Build history of the part. All positions in model axes, mm. A direction names the side the tool comes from. Round coordinates to 2 decimals unless told otherwise and drop trailing zeros. Write each loop counter-clockwise with the first axis right and the second up, starting at its lowest first coordinate (ties: lowest second). Pieces come first, ordered by that corner, then holes. Notation, with made-up numbers: (-7, 12.5) -> (47, 12.5) arc R18 cw to (47, 31.5) -> close; hole circle Ø2 at (25.25, 18). An arc over 180 degrees is marked (long way). One line per question, with ' | ' between items.
from build123d import *

# Parameters (mm, degrees)
F0_W     = 558.8
F0_H     = 330.2
F0_W_2   = 527.05
F0_H_2   = 298.45
F1_DEPTH = 25.4
F2_DEPTH = 19.05
F3_W     = 406.4
F3_H     = 209.55
F4_DEPTH = 19.05
F5_W     = 406.4
F5_H     = 15.875
F5_H_2   = 47.625
F6_DEPTH = 9.525
F8_DEPTH = 9.525


with BuildPart() as f1:
    # F0 (on Front) → F1 (new body)
    with BuildSketch(Plane.XZ):
        with Locations((-9.705722, 22.848336)):
            Rectangle(F0_W, F0_H)
        with Locations((-9.705722, 22.848336)):
            Rectangle(F0_W_2, F0_H_2, mode=Mode.SUBTRACT)
    extrude(amount=F1_DEPTH)

    # F0 (on Front) → F2 (join)
    with BuildSketch(Plane.XZ):
        with Locations((-9.705722, 22.848336)):
            Rectangle(F0_W_2, F0_H_2)
    extrude(amount=F2_DEPTH)

    # F3 (on face) → F4 (join)
    with BuildSketch(Plane.XZ):
        with Locations((-9.705722, 26.023336)):
            Rectangle(F3_W, F3_H)
    extrude(amount=-F4_DEPTH)

    # F5 (on face) → F6 (cut)
    with BuildSketch(Plane.XZ):
        with Locations((-9.705722, -134.314164)):
            Rectangle(F5_W, F5_H)
        with Locations((-9.705722, -102.564164)):
            Rectangle(F5_W, F5_H_2)
    extrude(amount=F6_DEPTH, mode=Mode.SUBTRACT)

    # F7 (on face) → F8 (join)
    with BuildSketch(Plane.XZ):
        Polygon((-50.980722, -126.376664), (31.569278, -126.376664), (31.996309, -78.751664), (31.569278, -78.751664), (-50.980722, -78.751664), align=None)
    extrude(amount=-F8_DEPTH)


solid = f1.part
(1) Slice it at A-A (z = 109.5). Write the cut outline in (x, y), then the cut area to 3 significant figures.
Calculated:
outline: (-289.11, -25.4) -> (-273.23, -25.4) -> (-273.23, -19.05) -> (253.82, -19.05) -> (253.82, -25.4) -> (269.69, -25.4) -> (269.69, 0) -> (193.49, 0) -> (193.49, 19.05) -> (-212.91, 19.05) -> (-212.91, 0) -> (-289.11, 0) -> close | area: 18,600 mm2
(2) Wall check: line 1 (X direction, y = 12, z = 117.5); line 2 (Y direction, x = 198.5, z = 53); line 3 (X direction, y = -19.5, z = 163.5). Give the ranges that are in metal, low to high. Write a range as from..to.
Calculated:
line 1: -212.91..193.49 | line 2: -19.05..0 | line 3: -289.11..-273.23, 253.82..269.69
(3) Slice it at C-C (x = -224.5). Write the cut outline in (y, z).
Calculated:
outline: (-25.4, -142.25) -> (0, -142.25) -> (0, 187.95) -> (-25.4, 187.95) -> (-25.4, 172.07) -> (-19.05, 172.07) -> (-19.05, -126.38) -> (-25.4, -126.38) -> close
(4) Drop flat-ended pins along their axis: pin 1 (3 mm diameter, centred on x = -189, y = 11.5, fed in from +Z); pin 2 (1.5 mm diameter, centred on x = -215.5, z = -76.5, fed in from -Y); pin 3 (24 mm diameter, centred on x = -25, z = -91, fed in from +Y) (3 decimals). Give the stop position or say it passes through.
Calculated:
pin 1: z = 130.8 | pin 2: y = -19.05 | pin 3: y = 9.525
(5) Mould opens along X. For faces 4 (the flat face through (193.494, 9, 25)), 5 (the flat face through (-13, -19.05, 25)), 6 (the flat face through (-14, -13, 187.948)) say: pulls with the +X half, pulls with the -X half, needs draft (parallel to the pull), parting line crosses it, or undercut.
Calculated:
face 4: pulls with the +X half | face 5: undercut | face 6: needs draft
(6) 3-axis set-ups, long thin cutter, end or side, ignore diameter. For faces 1 (the flat face through (-10, 0, -102)), 2 (the flat face through (-13, 9, 130.798)), 3 (the flat face through (-10, 9.525, -102)): which of +Z, -Z, +X, -X, +Y, -Y reach the whole face in a straight line?
Calculated:
face 1: -Z | face 2: +Z, +X, -X, +Y | face 3: -Z, +X, -X, +Y
(7) Slice it at B-B (x = 78). Write the cut outline in (y, z) (3 decimals).
Calculated:
outline: (-25.4, -142.252) -> (-9.525, -142.252) -> (-9.525, -78.752) -> (19.05, -78.752) -> (19.05, 130.798) -> (0, 130.798) -> (0, 187.948) -> (-25.4, 187.948) -> (-25.4, 172.073) -> (-19.05, 172.073) -> (-19.05, -126.377) -> (-25.4, -126.377) -> close
